from build123d import *

# Parameters (mm, degrees)
F1_DEPTH = 15
F2_W     = 19.2250516646
F2_H     = 20
F2_W_2   = 8
F3_DEPTH = 109.0935827289
F4_R     = 3.1
F5_DEPTH = 25
F6_DEPTH = 55.0010001


with BuildPart() as f1:
    # F0 (on Front) → F1 (new body, symmetric)
    with BuildSketch(Plane.XZ):
        with BuildLine():
            ThreePointArc((0, -12.5), (8.8388347648, -8.8388347648), (12.5, 0))
            ThreePointArc((12.5, 0), (8.8388347648, 8.8388347648), (0, 12.5))
            ThreePointArc((0, 12.5), (-12.5, 0), (0, -12.5))
        make_face()
        with BuildLine():
            ThreePointArc((0, 12.5), (8.8388347648, 8.8388347648), (12.5, 0))
            ThreePointArc((12.5, 0), (8.8388347648, -8.8388347648), (0, -12.5))
            Line((0, -12.5), (14.3338776639, -12.5))
            Line((14.3338776639, -12.5), (12.6173132409, 0))
            Line((12.6173132409, 0), (12.6173132409, 12.5))
            Line((12.6173132409, 12.5), (0, 12.5))
        make_face()
        with BuildLine():
            Line((12.6173132409, 52.036685962), (12.6173132409, 12.5))
            Line((12.6173132409, 12.5), (12.6173132409, 0))
            Line((12.6173132409, 0), (14.3338776639, -12.5))
            Line((14.3338776639, -12.5), (25.8819045103, -96.5925826289))
            add(Edge.make_bspline(
                [(25.8819045103, -96.5925826289), (72.6372622036, -84.0645222931), (12.6173132409, 52.036685962)],
                knots=[3.1415926536, 3.1415926536, 3.1415926536, 5.2016568498, 5.2016568498, 5.2016568498], degree=2, weights=[1, 0.514791327, 1]))
        make_face()
    extrude(amount=F1_DEPTH, both=True)

    # F2 (on face) → F3 (cut, through all)
    with BuildSketch(Plane.XY.offset(12.5)):
        with Locations((-9.6125258323, 0)):
            Rectangle(F2_W, F2_H)
        with Locations((4, 0)):
            Rectangle(F2_W_2, F2_H)
    extrude(amount=-F3_DEPTH, mode=Mode.SUBTRACT)

    # F4 (on face) → F5 (join)
    with BuildSketch(Plane.XZ.offset(15)):
        Circle(F4_R)
    extrude(amount=F5_DEPTH)

    # F6 (cut, through all): a face of the model
    f6_faces = [f1.faces().sort_by_distance(p)[0] for p in [
        (0, -40, 0),
    ]]
    extrude(f6_faces, amount=-F6_DEPTH, mode=Mode.SUBTRACT)


solid = f1.part
Verification items for the finished model (mm, model axes). A direction names the side the tool comes from. Give positions to 0.01 mm unless a question says otherwise; leave off trailing zeros.
1. Go/stop test with flat-tipped pins: P1, Ø10, axis at y = -3.5, z = -5.5, coming from the -X side; P2, Ø4.5, axis at x = 10, y = 7, coming from the -Z side; P3, Ø6, axis at x = 9, y = 0, coming from the +Z side. Record where each tip stops, or that it passes through.
Derived:
P1: stops at x = 8
P2: stops at z = -12.5
P3: stops at z = 12.5
2. Material ranges on probe 1 along Z at (x, y) = (0, 13.6); probe 2 along Z at (x, y) = (11, 9.5); probe 3 along X at (y, z) = (-8.5, -35), recorded low to high.
Derived:
probe 1: z = -12.5 to -3.1, 3.1 to 12.5
probe 2: z = -12.5 to 12.5
probe 3: x = 17.42 to 36.51
3. Tool access check on faces 1 (the cylindrical face through (-12.497, -12.535, 0.275)), 2 (the flat face through (9, 0, -12.5)), 3 (the flat face through (8, 0, 0)), 4 (the flat face through (9, 0, 12.5)). Record the directions out of +Z, -Z, +X, -X, +Y, -Y that give a thin tool (end or side, any length) a straight path to the whole face; none if there is none.
Derived:
face 1: -X, +Y, -Y
face 2: -Z, -X, +Y, -Y
face 3: +Z, -Z, -X
face 4: +Z, -X, +Y, -Y
4. Release check for a two-part mould opening along Y. For faces 5 (the flat face through (20, -15, -22)), 6 (the flat face through (-2, -10, -3)), 7 (the flat face through (12.617, 0, 33)), 8 (the flat face through (-2, 10, -3)) record: +Y half, -Y half, draft (parallel to the pull), parting line (faces both ways), or undercut.
Derived:
face 5: -Y half
face 6: undercut
face 7: draft
face 8: undercut
5. Cross-section at A-A on z = 0. Count the separate pieces of the cut face and the enclosed holes in it, and give its area (3 significant figures).
Derived:
separate pieces: 3
enclosed holes: 0
area: 803 mm2
